Read the model definition and answer for the solid it produces. Units are mm, in the model's axes. Face numbers are marked on the shaded views. Give positions to 0.01 mm unless a question says otherwise; leave off trailing zeros. Write each loop counter-clockwise with the first axis right and the second up, starting at its lowest first coordinate (ties: lowest second). Pieces come first, ordered by that corner, then holes. Notation, with made-up numbers: M 45.5,8 L 56.5,8 A13 cw 56.5,32 Z; hole C 57.25,1.5 d8. An arc over 180 degrees is marked long. Use a Markdown table: item, result. Add a question column.
Item 1: A cutting plane is placed at D-D on z = 24. Count the separate pieces of the cut face and the enclosed holes in it, then the cut area to 3 significant figures.
Item 2: A cutting plane is placed at C-C on x = -7. Determine the outline of the cut face in (y, z), then the cut area to 3 significant figures.
Item 3: Consider probe 1 along Y at (x, z) = (-8, 41.5); probe 2 along Y at (x, z) = (0.5, 39); probe 3 along Y at (x, z) = (15.5, 27.5). Determine where each line is inside the solid, lowest interval first. Write a range as [from, to].
Item 4: The mould has two halves that part along X. Classify the marked faces 1, 2 and 3: pulls with the +X half, pulls with the -X half, needs draft (parallel to the pull), parting line crosses it, or undercut.
Item 5: Given P1, Ø5, axis at x = -1, z = 43.5, coming from the +Y side; P2, Ø5, axis at y = 6, z = 38, coming from the -X side; P3, Ø1.1, axis at x = 15.5, y = -1.5, coming from the +Z side; P4, Ø4, axis at y = -6, z = 43, coming from the -X side, each flat-ended and moving along its own axis, determine where each tip first touches the part or whether it passes through.
Item 6: A cutting plane is placed at A-A on x = 0. Determine the outline of the cut face in (y, z) (3 decimals), then the cut area to 3 significant figures.
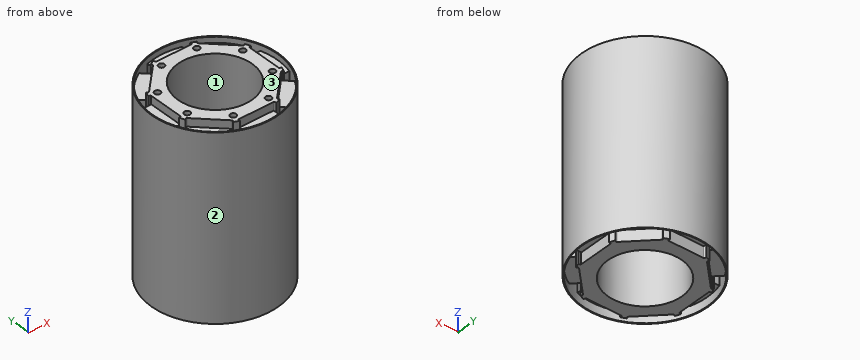
from build123d import *

# Parameters (mm, degrees)
SKETCH_1_R                       = 14.735
SKETCH_1_R_2                     = 10.005
EXTRUDE_1_DEPTH                  = 50.19
CUT_EXTRUDE_START                = 42
CUT_EXTRUDE_1_DEPTH              = 94.586205036
FILLET_1_R                       = 0.25
PATTERN_CIRCULAR_2_COUNT         = 8
FILLET_1_OF_PATTERN_CIRCULAR_2_R = 0.25
EXTRUDE_2_DEPTH                  = 45
PATTERN_CIRCULAR_4_COUNT         = 8
SKETCH_5_R                       = 17.12
SKETCH_5_R_2                     = 16.865
EXTRUDE_3_DEPTH                  = 48.91
PATTERN_CIRCULAR_6_COUNT         = 8


with BuildPart() as part:
    # 草图1 → 凸台-拉伸1 (new body)
    with BuildSketch(Plane.XY):
        with Locations(Location((0, 0, 0), (0, 0, 180))):
            Circle(SKETCH_1_R)
        with Locations(Location((0, 0, 0), (0, 0, 180))):
            Circle(SKETCH_1_R_2, mode=Mode.SUBTRACT)
    extrude(amount=EXTRUDE_1_DEPTH)

    # 草图3 → 切除-拉伸1 (cut)
    with BuildSketch(Plane(origin=(0, 0, 3), x_dir=(-1, 0, 0), z_dir=(0, 0, -1)).offset(CUT_EXTRUDE_START)):
        with BuildLine():
            Line((-4.9475, 13.879570193), (-4.9475, 13.31))
            Line((-4.9475, 13.31), (4.9475, 13.31))
            Line((4.9475, 13.31), (4.9475, 13.879570193))
            ThreePointArc((4.9475, 13.879570193), (0, 14.735), (-4.9475, 13.879570193))
        make_face()
    cut_extrude_1 = extrude(amount=-CUT_EXTRUDE_1_DEPTH, mode=Mode.SUBTRACT)

    # 圆角1
    fillet_1_edges = [part.edges().sort_by_distance(p)[0] for p in [
        (4.9475, 13.31, 25.095),
        (-4.9475, 13.31, 25.095),
    ]]
    fillet(fillet_1_edges, radius=FILLET_1_R)

    # 阵列(圆周)2: 切除-拉伸1 ×8 about axis
    pattern_circular_2_axis = Axis((0, 0, 0), (0, 0, 1))
    for i in range(1, PATTERN_CIRCULAR_2_COUNT):
        add(cut_extrude_1.rotate(pattern_circular_2_axis, i * 360 / PATTERN_CIRCULAR_2_COUNT), mode=Mode.SUBTRACT)

    # 圆角1 of 阵列(圆周)2
    fillet_1_of_pattern_circular_2_edges = [part.edges().sort_by_distance(p)[0] for p in [
        (-5.913180458, 12.910002058, 25.095),
        (-12.910002058, 5.913180458, 25.095),
        (-13.31, 4.9475, 25.095),
        (-13.31, -4.9475, 25.095),
        (-12.910002058, -5.913180458, 25.095),
        (-5.913180458, -12.910002058, 25.095),
        (-4.9475, -13.31, 25.095),
        (4.9475, -13.31, 25.095),
        (5.913180458, -12.910002058, 25.095),
        (12.910002058, -5.913180458, 25.095),
        (13.31, -4.9475, 25.095),
        (13.31, 4.9475, 25.095),
        (12.910002058, 5.913180458, 25.095),
        (5.913180458, 12.910002058, 25.095),
    ]]
    fillet(fillet_1_of_pattern_circular_2_edges, radius=FILLET_1_OF_PATTERN_CIRCULAR_2_R)

    # 草图4 → 凸台-拉伸2 (add)
    with BuildSketch(Plane(origin=(0, 0, 3), x_dir=(-1, 0, 0), z_dir=(0, 0, -1))):
        with BuildLine():
            Line((-4.6975, 13.31), (-4.6975, 16.197583732))
            ThreePointArc((-4.6975, 16.197583732), (0, 16.865), (4.6975, 16.197583732))
            Line((4.6975, 16.197583732), (4.6975, 13.31))
            Line((4.6975, 13.31), (-4.6975, 13.31))
        make_face()
    extrude_2 = extrude(amount=-EXTRUDE_2_DEPTH)

    # 阵列(圆周)4: 凸台-拉伸2 ×8 about axis
    pattern_circular_4_axis = Axis((0, 0, 0), (0, 0, 1))
    for i in range(1, PATTERN_CIRCULAR_4_COUNT):
        add(extrude_2.rotate(pattern_circular_4_axis, i * 360 / PATTERN_CIRCULAR_4_COUNT))

    # 草图5 → 凸台-拉伸3 (add)
    with BuildSketch(Plane(origin=(0, 0, 0.64), x_dir=(-1, 0, 0), z_dir=(0, 0, -1))):
        Circle(SKETCH_5_R)
        Circle(SKETCH_5_R_2, mode=Mode.SUBTRACT)
    extrude(amount=-EXTRUDE_3_DEPTH)

    # 草图9 → M2 螺纹孔2 (revolve, cut)
    with BuildSketch(Plane(origin=(-4.783542905, 11.548494156, 50.19), x_dir=(0, -1, 0), z_dir=(1, 0, 0))):
        Polygon((0, 0), (0, 5.680688495), (0.8, 5.2), (0.8, 0), align=None)
    hole_wizard_m2_2 = revolve(axis=Axis((-4.783542905, 11.548494156, 56.54), (0, 0, -1)), mode=Mode.SUBTRACT)

    # 阵列(圆周)6: M2 螺纹孔2 ×8 about axis
    pattern_circular_6_axis = Axis((0, 0, 0), (0, 0, 1))
    for i in range(1, PATTERN_CIRCULAR_6_COUNT):
        add(hole_wizard_m2_2.rotate(pattern_circular_6_axis, i * 360 / PATTERN_CIRCULAR_6_COUNT), mode=Mode.SUBTRACT)


solid = part.part
Filled in:
| question | item | result |
|---|---|---|
| 1 | separate pieces | 1 |
| 1 | enclosed holes | 9 |
| 1 | area | 555 mm² |
| 2 | outline | M -15.62,0.64 L -15.34,0.64 L -15.34,49.55 L -15.62,49.55 Z; M -13.64,3 L -11.82,3 L -11.82,0 L -7.15,0 L -7.15,50.19 L -11.82,50.19 L -11.82,48 L -13.64,48 Z; M 7.15,0 L 11.82,0 L 11.82,3 L 13.64,3 L 13.64,48 L 11.82,48 L 11.82,50.19 L 7.15,50.19 Z; M 15.34,0.64 L 15.62,0.64 L 15.62,49.55 L 15.34,49.55 Z |
| 2 | area | 660 mm² |
| 3 | probe 1 | [-15.14, -14.85], [-14.64, -6.01], [6.01, 14.64], [14.85, 15.14] |
| 3 | probe 2 | [-17.11, -9.99], [9.99, 17.11] |
| 3 | probe 3 | [-7.27, -6.65], [-4.7, 4.7], [6.65, 7.27] |
| 4 | face 1 | undercut |
| 4 | face 2 | parting line crosses it |
| 4 | face 3 | needs draft |
| 5 | P1 | y = 17.12 |
| 5 | P2 | x = -16.76 |
| 5 | P3 | z = 48 |
| 5 | P4 | x = -16.65 |
| 6 | outline | M -17.12,0.64 L -16.865,0.64 L -16.865,3 L -13.31,3 L -13.31,0 L -10.005,0 L -10.005,50.19 L -13.31,50.19 L -13.31,48 L -16.865,48 L -16.865,49.55 L -17.12,49.55 Z; M 10.005,0 L 13.31,0 L 13.31,3 L 16.865,3 L 16.865,0.64 L 17.12,0.64 L 17.12,49.55 L 16.865,49.55 L 16.865,48 L 13.31,48 L 13.31,50.19 L 10.005,50.19 Z |
| 6 | area | 677 mm² |
